from build123d import *

# Parameters (mm, degrees)
SKETCH3_W          = 6
SKETCH3_H          = 1
CUT_EXTRUDE1_DEPTH = 1.5


with BuildPart() as part:
    # Sketch2 → Revolve1 (revolve)
    with BuildSketch(Plane.XY):
        Polygon((0, -8.1), (2, -8.1), (2, 0), (3.6, 0), (3.6, 0.9), (3, 1.5), (3, 8.73125), (0, 8.73125), align=None)
    revolve(axis=Axis((0, 43.323370715, 0), (0, -1, 0)))

    # Sketch3 → Cut-Extrude1 (cut)
    with BuildSketch(Plane(origin=(0, 8.73125, 0), x_dir=(1, 0, 0), z_dir=(0, 1, 0))):
        Rectangle(SKETCH3_W, SKETCH3_H)
    extrude(amount=-CUT_EXTRUDE1_DEPTH, mode=Mode.SUBTRACT)


solid = part.part
For this review, take the finished solid that the model builds, in its own axes (mm). A direction names the side the tool comes from. Give positions to 0.01 mm unless a question says otherwise; leave off trailing zeros. Write each loop counter-clockwise with the first axis right and the second up, starting at its lowest first coordinate (ties: lowest second). Pieces come first, ordered by that corner, then holes. Notation, with made-up numbers: (67.5, 34.5) -> (94.5, 34.5) arc R4 cw to (94.5, 41.5) -> close; hole circle Ø7 at (12, -21.75). An arc over 180 degrees is marked (long way). Use CSV: the item, a comma, the result in double quotes.
Q1. Mouldability with a two-part tool opening along Z and no side actions: class faces 1 (the face through (0, 8.731, 1)), 2 (the face through (2.86, 5.17, 0.9)), 3 (the face through (0, 7.231, 0)) as pulls with the +Z half, pulls with the -Z half, needs draft (parallel to the pull), parting line crosses it, or undercut.
Conclusion:
face 1,"needs draft"
face 2,"parting line crosses it"
face 3,"undercut"
Q2. Take a section at A-A, the plane x = 0. Write out the cut boundary in (y, z).
Conclusion:
outline,"(-8.1, -2) -> (0, -2) -> (0, -3.6) -> (0.9, -3.6) -> (1.5, -3) -> (8.73, -3) -> (8.73, -0.5) -> (7.23, -0.5) -> (7.23, 0.5) -> (8.73, 0.5) -> (8.73, 3) -> (1.5, 3) -> (0.9, 3.6) -> (0, 3.6) -> (0, 2) -> (-8.1, 2) -> close"
Q3. For P1, Ø1, axis at x = 2.5, y = 3.5, coming from the +Z side; P2, Ø3, axis at y = -2.5, z = -2, coming from the -X side; P3, Ø1.2, axis at x = -1, y = 8, coming from the -Z side, all flat-tipped, find the tip position at first contact; note any pin that passes through.
Conclusion:
P1,"z = 2.24"
P2,"x = -1.94"
P3,"z = -2.97"
Q4. Tool access review of faces 4 (the face through (0, 8, -0.5)), 5 (the face through (0, -8.1, 0)), 6 (the face through (-2, 0, -2)): name each direction out of +Z, -Z, +X, -X, +Y, -Y from which nothing blocks a thin tool from reaching the whole face with its end or side.
Conclusion:
face 4,"+X, -X, +Y"
face 5,"+Z, -Z, +X, -X, -Y"
face 6,"-Y"
Q5. To check wall thickness, follow probe 1 along Y at (x, z) = (0.75, -2.25); probe 2 along Y at (x, z) = (1.25, 0); probe 3 along Z at (x, y) = (-0.5, 6.5). State the ranges of each line that lie inside material, in increasing order. Write a range as [from, to].
Conclusion:
probe 1,"[0, 8.73]"
probe 2,"[-8.1, 7.23]"
probe 3,"[-2.96, 2.96]"
Q6. Take a section at C-C, the plane y = -1.25. Write out the cut boundary in (x, z), then the cut area to 3 significant figures.
Conclusion:
outline,"circle Ø4 at (0, 0)"
area,"12.6 mm2"
Q7. Take a section at D-D, the plane y = 7. Write out the cut boundary in (x, z).
Conclusion:
outline,"circle Ø6 at (0, 0)"
Q8. Take a section at B-B, the plane z = 0. Write out the cut boundary in (x, y), then the cut area to 3 significant figures.
Conclusion:
outline,"(-3.6, 0) -> (-2, 0) -> (-2, -8.1) -> (2, -8.1) -> (2, 0) -> (3.6, 0) -> (3.6, 0.9) -> (3, 1.5) -> (3, 7.23) -> (-3, 7.23) -> (-3, 1.5) -> (-3.6, 0.9) -> close"
area,"77.2 mm2"
